Design review of the part built by this model. Coordinates are the model's own, in mm. Give positions to 0.01 mm unless a question says otherwise; leave off trailing zeros. Loops run counter-clockwise (first coordinate to the right, second up) from the corner with the lowest first, then second, coordinate; pieces in that order, holes last. Notation, with made-up numbers: (81.25, 58) -> (114.25, 58) arc R13 ccw to (114.25, 83) -> close; hole circle Ø11 at (22.25, 88). An arc over 180 degrees is marked (long way). Use a Markdown table: item, result. Add a question column.
1. Add section A-A (z = 33.5). State the section outline as (x, y) points.
2. To check wall thickness, follow line 1 (X direction, y = 87.5, z = 38.5); line 2 (X direction, y = 59.5, z = -84); line 3 (Y direction, x = 91.5, z = -45). State the ranges of each line that lie inside material, in increasing order.
3. Add section B-B (y = 88). State the section outline as (x, z) points.
```python
from build123d import *

# Parameters (mm, degrees)
SKETCH_1_W      = 200
SKETCH_1_H      = 200
EXTRUDE_1_DEPTH = 100
CHAMFER_1_SIZE  = 18


with BuildPart() as part:
    # 草图1 → 凸台-拉伸1 (new, symmetric)
    with BuildSketch(Plane.XY):
        Rectangle(SKETCH_1_W, SKETCH_1_H)
    extrude(amount=EXTRUDE_1_DEPTH, both=True)

    # 倒角1
    chamfer_1_edges = [part.edges().sort_by_distance(p)[0] for p in [
        (-100, 0, 100),
        (0, -100, 100),
        (100, 0, 100),
        (0, -100, -100),
        (-100, 0, -100),
        (0, 100, -100),
        (100, 0, -100),
        (100, -100, 0),
        (-100, -100, 0),
        (-100, 100, 0),
        (100, 100, 0),
        (0, 100, 100),
    ]]
    chamfer(chamfer_1_edges, length=CHAMFER_1_SIZE)


solid = part.part
```
Taken from the geometry:
| question | item | result |
|---|---|---|
| 1 | outline | (-100, -82) -> (-82, -100) -> (82, -100) -> (100, -82) -> (100, 82) -> (82, 100) -> (-82, 100) -> (-100, 82) -> close |
| 2 | line 1 | x = -94.5 to 94.5 |
| 2 | line 2 | x = -98 to 98 |
| 2 | line 3 | y = -90.5 to 90.5 |
| 3 | outline | (-94, -82) -> (-82, -94) -> (82, -94) -> (94, -82) -> (94, 82) -> (82, 94) -> (-82, 94) -> (-94, 82) -> close |
